from build123d import *

# Parameters (mm, degrees)
F0_R     = 6
F0_W     = 12
F0_H     = 10
F0_R_2   = 2.75
F1_DEPTH = 2
F2_DEPTH = 15
F3_W     = 4
F3_H     = 3.5
F6_DEPTH = 6


with BuildPart() as f1:
    # F0 (on Top) → F1 (new body)
    with BuildSketch(Plane.XY):
        with BuildLine():
            Line((-25.5, 35), (-45, 35))
            ThreePointArc((-45, 35), (-48.5355339059, 33.5355339059), (-50, 30))
            Line((-50, 30), (-50, -30))
            ThreePointArc((-50, -30), (-48.5355339059, -33.5355339059), (-45, -35))
            Line((-45, -35), (-35.5, -35))
            Line((-35.5, -35), (-25.5, 35))
        make_face()
        with Locations((-42, -20)):
            Circle(F0_R, mode=Mode.SUBTRACT)
        with Locations((-42, 25)):
            Circle(F0_R, mode=Mode.SUBTRACT)
        Polygon((25.5, 35), (-25.5, 35), (-35.5, -35), (35.5, -35), align=None)
        with Locations((0, -17)):
            Rectangle(F0_W, F0_H, mode=Mode.SUBTRACT)
        with BuildLine():
            Line((45, 35), (25.5, 35))
            Line((25.5, 35), (35.5, -35))
            Line((35.5, -35), (45, -35))
            ThreePointArc((45, -35), (48.5355339059, -33.5355339059), (50, -30))
            Line((50, -30), (50, 30))
            ThreePointArc((50, 30), (48.5355339059, 33.5355339059), (45, 35))
        make_face()
        with Locations((42, -20)):
            Circle(F0_R, mode=Mode.SUBTRACT)
        with Locations((42, 25)):
            Circle(F0_R, mode=Mode.SUBTRACT)
        with Locations((-42, 25)):
            Circle(F0_R)
        with Locations((-42, 25)):
            Circle(F0_R_2, mode=Mode.SUBTRACT)
        with Locations((-42, -20)):
            Circle(F0_R)
        with Locations((-42, -20)):
            Circle(F0_R_2, mode=Mode.SUBTRACT)
        with Locations((42, -20)):
            Circle(F0_R)
        with Locations((42, -20)):
            Circle(F0_R_2, mode=Mode.SUBTRACT)
        with Locations((42, 25)):
            Circle(F0_R)
        with Locations((42, 25)):
            Circle(F0_R_2, mode=Mode.SUBTRACT)
    extrude(amount=-F1_DEPTH)

    # F0 (on Top) → F2 (join)
    with BuildSketch(Plane.XY):
        with BuildLine():
            Line((-25.5, 35), (-45, 35))
            ThreePointArc((-45, 35), (-48.5355339059, 33.5355339059), (-50, 30))
            Line((-50, 30), (-50, -30))
            ThreePointArc((-50, -30), (-48.5355339059, -33.5355339059), (-45, -35))
            Line((-45, -35), (-35.5, -35))
            Line((-35.5, -35), (-25.5, 35))
        make_face()
        with Locations((-42, -20)):
            Circle(F0_R, mode=Mode.SUBTRACT)
        with Locations((-42, 25)):
            Circle(F0_R, mode=Mode.SUBTRACT)
        with BuildLine():
            Line((45, 35), (25.5, 35))
            Line((25.5, 35), (35.5, -35))
            Line((35.5, -35), (45, -35))
            ThreePointArc((45, -35), (48.5355339059, -33.5355339059), (50, -30))
            Line((50, -30), (50, 30))
            ThreePointArc((50, 30), (48.5355339059, 33.5355339059), (45, 35))
        make_face()
        with Locations((42, -20)):
            Circle(F0_R, mode=Mode.SUBTRACT)
        with Locations((42, 25)):
            Circle(F0_R, mode=Mode.SUBTRACT)
    extrude(amount=F2_DEPTH)

    # F4: sweep along a path in F4_path
    with BuildLine(Plane(origin=(-35.5, -35, 15), x_dir=(-0.1414213562, -0.9899494937, 0), z_dir=(0.9899494937, -0.1414213562, 0))) as f4_path:
        Line((0, 0), (-70.7106781187, 0))
    # F3 (on face) → F4 (sweep)
    with BuildSketch(Plane.XZ.offset(35)):
        with Locations((-33.5, 13.25)):
            Rectangle(F3_W, F3_H)
    sweep(path=f4_path.line)

    # F5: sweep along a path in F5_path
    with BuildLine(Plane(origin=(35.5, -35, 15), x_dir=(0.1414213562, -0.9899494937, 0), z_dir=(0.9899494937, 0.1414213562, 0))) as f5_path:
        Line((0, 0), (-70.7106781187, 0))
    # F3 (on face) → F5 (sweep)
    with BuildSketch(Plane.XZ.offset(35)):
        with Locations((33.5, 13.25)):
            Rectangle(F3_W, F3_H)
    sweep(path=f5_path.line)

    # F0 (on Top) → F6 (join)
    with BuildSketch(Plane.XY):
        with Locations((-42, -20)):
            Circle(F0_R)
        with Locations((-42, -20)):
            Circle(F0_R_2, mode=Mode.SUBTRACT)
        with Locations((-42, 25)):
            Circle(F0_R)
        with Locations((-42, 25)):
            Circle(F0_R_2, mode=Mode.SUBTRACT)
        with Locations((42, 25)):
            Circle(F0_R)
        with Locations((42, 25)):
            Circle(F0_R_2, mode=Mode.SUBTRACT)
        with Locations((42, -20)):
            Circle(F0_R)
        with Locations((42, -20)):
            Circle(F0_R_2, mode=Mode.SUBTRACT)
    extrude(amount=F6_DEPTH)


solid = f1.part
Input: part model. Units: mm. Frame: model coordinates. A direction names the side the tool comes from. Give positions to 0.01 mm unless a question says otherwise; leave off trailing zeros. Write each loop counter-clockwise with the first axis right and the second up, starting at its lowest first coordinate (ties: lowest second). Pieces come first, ordered by that corner, then holes. Notation, with made-up numbers: M 29,45.5 L 70,45.5 A22 cw 70,54.5 Z; hole C 60.25,39 d5. An arc over 180 degrees is marked long. Use one line per item in the form item = value.
1. First-contact query: P1, Ø3.5, axis at x = 42, y = 25, coming from the +Z side; P2, Ø3.5, axis at x = -41.5, y = -18.5, coming from the +Z side; P3, Ø4, axis at x = 0, y = -3, coming from the +Z side. Flat tips, straight axial feed; report the tip coordinate or a pass-through.
Outcome:
P1 = through
P2 = 6
P3 = 0
2. Reachability of faces 1 (the face through (6, -17, -1)), 2 (the face through (30.43, 0.49, 5.67)), 3 (the face through (36, -20, 10)) from +Z, -Z, +X, -X, +Y, -Y: full face, straight path, thin tool, end or side. Return the list, or none.
Outcome:
face_1 = +Z, -Z
face_2 = -Y
face_3 = +Z
3. Cut plane C-C on x = -42. Return loops of the section in (y, z).
Outcome:
outline = M -35,-2 L -22.75,-2 L -22.75,6 L -26,6 L -26,15 L -35,15 Z; M -17.25,-2 L 22.25,-2 L 22.25,6 L 19,6 L 19,15 L -14,15 L -14,6 L -17.25,6 Z; M 27.75,-2 L 35,-2 L 35,15 L 31,15 L 31,6 L 27.75,6 Z
4. Ray query, L1, parallel to Y at x = -42, z = 3.75; L2, parallel to Y at x = 42, z = 8.25; L3, parallel to X at y = 28, z = 8. Return the intervals inside material, ascending.
Outcome:
L1 = -35 to -22.75, -17.25 to 22.25, 27.75 to 35
L2 = -35 to -26, -14 to 19, 31 to 35
L3 = -50 to -47.2, -36.8 to -26.5, 26.5 to 36.8, 47.2 to 50
5. Cut plane B-B on x = -3.5. Return loops of the section in (y, z), and give its area (3 significant figures).
Outcome:
outline = M -35,-2 L -22,-2 L -22,0 L -35,0 Z; M -12,-2 L 35,-2 L 35,0 L -12,0 Z
area = 120 mm²
6. Cut plane D-D on y = -20. State how many separate pieces and enclosed holes the cut face has, and give its area (3 significant figures).
Outcome:
separate_pieces = 4
enclosed_holes = 0
area = 399 mm²
7. Mould query, pull axis Z, two halves, no side actions, for faces 4 (the face through (-30.57, -0.49, 5.67)), 5 (the face through (-48, 25, 10)), 6 (the face through (-1, 0, -2)). Classes: released by +Z, released by -Z, zero draft, split by the parting line, or undercut.
Outcome:
face_4 = undercut
face_5 = zero draft
face_6 = released by -Z
8. Cut plane A-A on z = 1.75. Return loops of the section in (x, y), and give its area (3 significant figures).
Outcome:
outline = M -50,-30 A5 ccw -45,-35 L -35.5,-35 L -25.5,35 L -45,35 A5 ccw -50,30 Z; M 25.5,35 L 35.5,-35 L 45,-35 A5 ccw 50,-30 L 50,30 A5 ccw 45,35 Z; hole C -42,-20 d5.5; hole C -42,25 d5.5; hole C 42,-20 d5.5; hole C 42,25 d5.5
area = 2,610 mm²
